Read the model definition and answer for the solid it produces. Units are mm, in the model's axes. A direction names the side the tool comes from. Round coordinates to 2 decimals unless told otherwise and drop trailing zeros. Order: outer loops, then holes, each group sorted by start corner. A loop starts at its lowest first (then second) coordinate and runs counter-clockwise, first axis right, second up. Notation, with made-up numbers: (-36.75, 56.25) - (-13.75, 56.25) arc R9 ccw to (-13.75, 60.25) - close; hole circle Ø7 at (-28.75, -32). An arc over 180 degrees is marked (long way). One line per question, with ' | ' between items. Start each with the question number.
1) The part is cut by section A-A, the plane y = 15.75. Give the vertices of the cut face in (x, z).
2) For faces 1 (the flat face through (-22.54, 16.85, -15.34)), 2 (the flat face through (-6.5, 0, 6.5)), determine the directions among +Z, -Z, +X, -X, +Y, -Y from which every point of the face is accessible in a straight line to the end or side of a thin tool.
3) Straight lines are drawn through the part: line 1 (X direction, y = 2.15, z = 0); line 2 (Y direction, x = 15, z = 1.5); line 3 (Z direction, x = -26.5, y = 14). For each, find the intervals that lie inside material, in ascending order. Write a range as from..to.
4) The part is cut by section D-D, the plane z = -19. Give the vertices of the cut face in (x, y), plus the area to 3 significant figures.
5) Flat-ended cylindrical pins translate along their axes: pin 1 (8 mm diameter, centred on x = 16, z = -1.5, fed in from -Y); pin 2 (1 mm diameter, centred on y = 21, z = -6.5, fed in from -X); pin 3 (12 mm diameter, centred on x = -20, y = 9.5, fed in from -Z); pin 4 (2.5 mm diameter, centred on x = -23.5, z = -10.5, fed in from +Y). Find the tip coordinate at first contact, or state that the pin passes through.
6) The part is cut by section B-B, the plane z = -3. Give the vertices of the cut face in (x, y).
7) The part is cut by section C-C, the plane x = 0. Give the vertices of the cut face in (y, z).
8) The mould has two halves that part along X. Classify faces 3 (the cylindrical face through (30.736, 13.804, -4.036)), 4 (the flat face through (12, 28, -23)), 5 (the flat face through (0, 3, 11)): pulls with the +X half, pulls with the -X half, needs draft (parallel to the pull), parting line crosses it, or undercut.
from build123d import *

# Parameters (mm, degrees)
SKETCH1_R           = 31
BOSS_EXTRUDE1_DEPTH = 3
SKETCH2_R           = 31
SKETCH2_R_2         = 25.6
BOSS_EXTRUDE2_DEPTH = 25
SKETCH4_R           = 9
CUT_EXTRUDE1_DEPTH  = 51.467811524
CAVITY1_START       = 6
CAVITY1_DEPTH       = 22


# Read off the part's stored shape, not the designer's step: Cavity1
with BuildPart() as part:
    # Sketch1 → Boss-Extrude1 (new body)
    with BuildSketch(Plane(origin=(0, 0, 0), x_dir=(1, 0, 0), z_dir=(0, 1, 0))):
        with Locations(Location((0, 0, 0), (0, 0, 270))):
            Circle(SKETCH1_R)
    extrude(amount=BOSS_EXTRUDE1_DEPTH)

    # Sketch2 → Boss-Extrude2 (add)
    with BuildSketch(Plane(origin=(0, 3, 0), x_dir=(1, 0, 0), z_dir=(0, 1, 0))):
        with Locations(Location((0, 0, 0), (0, 0, 270))):
            Circle(SKETCH2_R)
        with Locations(Location((0, 0, 0), (0, 0, 270))):
            Circle(SKETCH2_R_2, mode=Mode.SUBTRACT)
    extrude(amount=BOSS_EXTRUDE2_DEPTH)

    # Sketch4 → Cut-Extrude1 (cut, through all)
    with BuildSketch(Plane(origin=(0, 3, 0), x_dir=(1, 0, 0), z_dir=(0, 1, 0))):
        with Locations(Location((0, 0, 0), (0, 0, 270))):
            Circle(SKETCH4_R)
    extrude(amount=-CUT_EXTRUDE1_DEPTH, mode=Mode.SUBTRACT)

    # Cavity1 outline → Cavity1 (cut)
    with BuildSketch(Plane(origin=(0, 0, 0), x_dir=(1, 0, 0), z_dir=(0, 1, 0)).offset(CAVITY1_START)):
        with BuildLine():
            ThreePointArc((-2.295619613, -28.894863729), (6.673679903, -28.599701426), (14.847278424, -24.894604691))
            Line((14.847278424, -24.894604691), (12.866647777, -22.131637422))
            ThreePointArc((12.866647777, -22.131637422), (5.817422257, -24.930254677), (-1.742424083, -25.540633475))
            Line((-1.742424083, -25.540633475), (-2.295619613, -28.894863729))
        make_face()
        with BuildLine():
            Line((-28.982999292, -0.410817947), (-25.599884123, -0.077025125))
            ThreePointArc((-25.599884123, -0.077025125), (-24.498945002, 7.427091879), (-21.247625377, 14.279300258))
            Line((-21.247625377, 14.279300258), (-23.875876221, 16.435496767))
            ThreePointArc((-23.875876221, 16.435496767), (-28.104907927, 8.52027438), (-28.982999292, -0.410817947))
        make_face()
        with BuildLine():
            ThreePointArc((12.733236347, 22.208662547), (18.681522745, 17.503162798), (22.99004946, 11.261333217))
            Line((22.99004946, 11.261333217), (26.171495835, 12.459366962))
            ThreePointArc((26.171495835, 12.459366962), (21.431228024, 20.079427046), (14.135720867, 25.305422638))
            Line((14.135720867, 25.305422638), (12.733236347, 22.208662547))
        make_face()
    extrude(amount=CAVITY1_DEPTH, mode=Mode.SUBTRACT)


solid = part.part
Values:
1) outline: circle Ø62 at (0, 0); hole (-28.98, 0.41) arc R23 ccw to (-23.88, -16.44) - (-21.25, -14.28) arc R25.6 ccw to (12.73, -22.21) - (14.14, -25.31) arc R23 ccw to (26.17, -12.46) - (22.99, -11.26) arc R25.6 ccw to (12.87, 22.13) - (14.85, 24.89) arc R23 ccw to (-2.3, 28.89) - (-1.74, 25.54) arc R25.6 ccw to (-25.6, 0.08) - close
2) face 1: +Y | face 2: +Z, -Z, +X, -X, -Y
3) line 1: x = -31..-9, 9..31 | line 2: y = 0..3 | line 3: z = -16.09..-12.46, 0.17..16.09
4) outline: (-24.49, 0) - (24.49, 0) - (24.49, 28) - (22.38, 28) - (22.38, 6) - (17.16, 6) - (17.16, 3) - (-17.16, 3) - (-17.16, 28) - (-24.49, 28) - close | area: 399 mm^2
5) pin 1: stops at y = 0 | pin 2: stops at x = -30.41 | pin 3: stops at z = -27.66 | pin 4: stops at y = 6
6) outline: (-30.85, 0) - (-8.49, 0) - (-8.49, 3) - (-25.42, 3) - (-25.42, 6) - (-29.07, 6) - (-29.07, 28) - (-30.85, 28) - close; (8.49, 0) - (30.85, 0) - (30.85, 28) - (25.42, 28) - (25.42, 3) - (8.49, 3) - close
7) outline: (0, -31) - (28, -31) - (28, -25.6) - (3, -25.6) - (3, -9) - (0, -9) - close; (0, 9) - (3, 9) - (3, 25.6) - (6, 25.6) - (6, 29.16) - (28, 29.16) - (28, 31) - (0, 31) - close
8) face 3: parting line crosses it | face 4: needs draft | face 5: undercut
